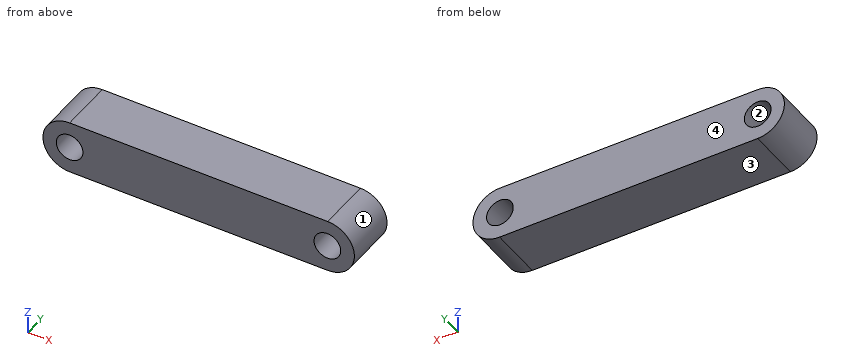
Solid Edge part; units mm, degrees
sketch "Sketch1" plane through (0, 0, 0) normal (0, -1, 0) x (1, 0, 0)
  arc A0 (-24.145, -5) -> (-24.145, 5) centre (-24.145, 0) cw
  line L0 (-24.145, 5) -> (24.2019, 5)
  arc A1 (24.2019, 5) -> (24.2019, -5) centre (24.2019, 0) cw
  line L1 (24.2019, -5) -> (-24.145, -5)
  circle A2 centre (24.145, 0) radius 2.5
  circle A3 centre (-24.145, 0) radius 2.5
  dimension "D1" = 24.145
extrude "Protrusion1" add sketch "Sketch1" along normal mid plane 10
The model under review builds one solid part; all positions refer to its coordinate system, in mm. Face numbers are marked on the shaded views. Round coordinates to 2 decimals unless told otherwise and drop trailing zeros. Write each loop counter-clockwise with the first axis right and the second up, starting at its lowest first coordinate (ties: lowest second). Pieces come first, ordered by that corner, then holes.
(1) Mouldability with a two-part tool opening along Z and no side actions: class the marked faces 1, 2, 3 and 4 as +Z half, -Z half, draft (parallel to the pull), parting line (faces both ways), or undercut.
(2) We need section B-B on y = -2.25. Give the boundary of the cut face in (x, z) (3 decimals), and give its area (3 significant figures).
(3) Wall thickness on L1, parallel to X at y = -4.25, z = 2 (3 decimals); L2, parallel to Z at x = -25, y = -1.25; L3, parallel to X at y = -3.75, z = -0.75: over which ranges is each line inside the solid? List them lowest first.
(4) We need section A-A on z = 0. Give the boundary of the cut face in (x, y) (3 decimals), and give its area (3 significant figures).
Findings below:
1. face 1: parting line
1. face 2: undercut
1. face 3: -Z half
1. face 4: draft
2. outline: (-24.145, -5) - (24.202, -5) arc R5 ccw to (24.202, 5) - (-24.145, 5) arc R5 ccw to start; hole circle Ø5 at (-24.145, 0); hole circle Ø5 at (24.145, 0)
2. area: 523 mm2
3. L1: x = -28.728 to -25.645, -22.645 to 22.645, 25.645 to 28.784
3. L2: z = -4.93 to -2.35, 2.35 to 4.93
3. L3: x = -29.09 to -26.53, -21.76 to 21.76, 26.53 to 29.15
4. outline: (-29.145, -5) - (-26.645, -5) - (-26.645, 5) - (-29.145, 5) - close; (-21.645, -5) - (21.645, -5) - (21.645, 5) - (-21.645, 5) - close; (26.645, -5) - (29.202, -5) - (29.202, 5) - (26.645, 5) - close
4. area: 483 mm2
